Can you work these out from the model? Positions are in its coordinate system, mm. A direction names the side the tool comes from. Round coordinates to 2 decimals unless told otherwise and drop trailing zeros. Order: outer loops, then holes, each group sorted by start corner. A loop starts at its lowest first (then second) coordinate and runs counter-clockwise, first axis right, second up. Notation, with made-up numbers: (34, 21) - (72, 21) arc R32 ccw to (72, 51) - close; hole circle Ø5 at (19, 54.5). An arc over 180 degrees is marked (long way). Write item = value, one per line.
from build123d import *

# Parameters (mm, degrees)
DODANIE_WYCI_GNI_CIE1_DEPTH = 10
SZKIC2_R                    = 1.55
WYTNIJ_WYCI_GNI_CIE1_DEPTH  = 10


with BuildPart() as part:
    # Szkic1 → Dodanie-wyciągnięcie1 (new body)
    with BuildSketch(Plane.XY):
        with BuildLine():
            Line((650.135201584, -439.296174139), (667.497764869, -439.296174139))
            ThreePointArc((667.497764869, -439.296174139), (681.639900492, -433.438309763), (687.497764869, -419.296174139))
            Line((687.497764869, -419.296174139), (687.49242436, -412.499258381))
            Line((687.49242436, -412.499258381), (687.49242436, -407.696233576))
            ThreePointArc((687.49242436, -407.696233576), (685.588618438, -403.100039498), (680.99242436, -401.196233576))
            Line((680.99242436, -401.196233576), (678.99242436, -401.196233576))
            ThreePointArc((678.99242436, -401.196233576), (676.99242436, -403.196233576), (678.99242436, -405.196233576))
            ThreePointArc((678.99242436, -405.196233576), (680.760191313, -405.928466623), (681.49242436, -407.696233576))
            Line((681.49242436, -407.696233576), (681.49242436, -410.309613134))
            add(Edge.make_bspline(
                [(672.570535689, -415.296173961), (680.339252513, -414.463379514), (681.49242436, -410.309613134)],
                knots=[0, 0, 0, 0.645201515, 0.645201515, 0.645201515], degree=2))
            Line((672.570535689, -415.296173961), (655.885201584, -415.296173961))
            ThreePointArc((655.885201584, -415.296173961), (653.056774459, -416.467746836), (651.885201584, -419.296173961))
            Line((651.885201584, -419.296173961), (651.885201584, -425.296174139))
            ThreePointArc((651.885201584, -425.296174139), (651.592308365, -426.00328092), (650.885201584, -426.296174139))
            Line((650.885201584, -426.296174139), (647.885201584, -426.296174139))
            Line((647.885201584, -426.296174139), (586.55506807, -426.296174139))
            Line((586.55506807, -426.296174139), (586.55506807, -419.296173961))
            ThreePointArc((586.55506807, -419.296173961), (585.383495195, -416.467746836), (582.55506807, -415.296173961))
            Line((582.55506807, -415.296173961), (567.724994048, -415.296173961))
            add(Edge.make_bspline(
                [(567.724994048, -415.296173961), (559.956277225, -414.463379514), (558.803105378, -410.309613134)],
                knots=[0, 0, 0, 0.645201515, 0.645201515, 0.645201515], degree=2))
            Line((558.803105378, -410.309613134), (558.803105378, -407.696233576))
            ThreePointArc((558.803105378, -407.696233576), (559.535338425, -405.928466623), (561.303105378, -405.196233576))
            ThreePointArc((561.303105378, -405.196233576), (563.303105378, -403.196233576), (561.303105378, -401.196233576))
            Line((561.303105378, -401.196233576), (559.303105378, -401.196233576))
            ThreePointArc((559.303105378, -401.196233576), (554.7069113, -403.100039498), (552.803105378, -407.696233576))
            Line((552.803105378, -407.696233576), (552.803105378, -412.499258381))
            Line((552.803105378, -412.499258381), (552.803105378, -419.296174139))
            ThreePointArc((552.803105378, -419.296174139), (558.660969754, -433.438309763), (572.803105378, -439.296174139))
            Line((572.803105378, -439.296174139), (588.30506807, -439.296174139))
            Line((588.30506807, -439.296174139), (650.135201584, -439.296174139))
        make_face()
    extrude(amount=DODANIE_WYCI_GNI_CIE1_DEPTH)

    # Szkic2 → Wytnij-wyciągnięcie1 (cut)
    with BuildSketch(Plane.XY.offset(10)):
        with Locations((631.130089997, -432.296174368)):
            Circle(SZKIC2_R)
        with Locations((607.164083377, -432.296174368)):
            Circle(SZKIC2_R)
    extrude(amount=-WYTNIJ_WYCI_GNI_CIE1_DEPTH, mode=Mode.SUBTRACT)


solid = part.part
(1) If I drill on line 1 (Y direction, x = 607, z = 3.5); line 2 (X direction, y = -419, z = 1.25); line 3 (Y direction, x = 612, z = 1.5), over which ranges is the centre line in solid material (lowest first)? Write a range as from..to.
Computed:
line_1 = -439.3..-433.84, -430.75..-426.3
line_2 = 552.8..586.54, 651.9..687.5
line_3 = -439.3..-426.3
(2) Thinking about a two-plate mould opening in Y: for faces 4 (the face through (685.64, -403.15, 4.93)), 5 (the face through (586.555, -423, 5)), 6 (the face through (676.993, -403.152, 4.93)), which applies, +Y half, -Y half, draft (parallel to the pull), parting line (faces both ways), or undercut?
Computed:
face_4 = +Y half
face_5 = draft
face_6 = undercut
(3) If we section it at C-C (y = -422.5): Write out the boundary of the cut face in (x, z).
Computed:
outline = (553.06, 0) - (586.56, 0) - (586.56, 10) - (553.06, 10) - close; (651.89, 0) - (687.24, 0) - (687.24, 10) - (651.89, 10) - close
(4) If we section it at A-A (y = -417.5): Write out the boundary of the cut face in (x, z), plus the area to 3 significant figures.
Computed:
outline = (552.8, 0) - (586.13, 0) - (586.13, 10) - (552.8, 10) - close; (652.31, 0) - (687.5, 0) - (687.5, 10) - (652.31, 10) - close
area = 685 mm^2
(5) If we section it at B-B (x = 589.5): Write out the boundary of the cut face in (y, z), plus the area to 3 significant figures.
Computed:
outline = (-439.3, 0) - (-426.3, 0) - (-426.3, 10) - (-439.3, 10) - close
area = 130 mm^2
(6) On a 3-axis mill with a long thin cutter (end or side, diameter ignored), from which of +Z, -Z, +X, -X, +Y, -Y can I reach the whole of each face in a straight line? I mean faces 1 (the face through (558.506, -433.282, 4.93)), 2 (the face through (559.516, -405.948, 4.93)), 3 (the face through (585.414, -416.499, 4.93)). Say none if no direction works.
Computed:
face_1 = +Z, -Z, -X, -Y
face_2 = +Z, -Z
face_3 = +Z, -Z, +Y
(7) If we section it at D-D (z = 7.5): State how many separate pieces and enclosed holes the cut face has, plus the area to 3 significant figures.
Computed:
separate_pieces = 1
enclosed_holes = 2
area = 2,530 mm^2
(8) Will these pins go through, and if not, where does the flat tip stop? P1, Ø5, axis at x = 659, z = 5.5, coming from the +Y side; P2, Ø4, axis at y = -427, z = 1, coming from the -X side; P3, Ø5.5, axis at y = -410, z = 3, coming from the +X side.
Computed:
P1 = -415.3
P2 = 553.63
P3 = 687.49
